Verification items for the finished model (mm, model axes). Give positions to 0.01 mm unless a question says otherwise; leave off trailing zeros. Loops run counter-clockwise (first coordinate to the right, second up) from the corner with the lowest first, then second, coordinate; pieces in that order, holes last. Notation, with made-up numbers: M 76.25,86.5 L 125.25,86.5 A10 ccw 125.25,99.5 Z; hole C -20.5,-19 d4. An arc over 180 degrees is marked long. Put each result on its own line as item: value. Start each with the question number.
from build123d import *

# Parameters (mm, degrees)
SKETCH_1_W          = 7.5
SKETCH_1_H          = 150
CUT_EXTRUDE_1_DEPTH = 1


with BuildPart() as part:
    # Sketch 1 → Revolve 1 (revolve)
    with BuildSketch(Plane.XY):
        Rectangle(SKETCH_1_W, SKETCH_1_H)
    revolve(axis=Axis((3.75, 75, 0), (0, -1, 0)))

    # Sketch 2 → Cut-Extrude 1 (cut, symmetric)
    with BuildSketch(Plane.XY):
        Polygon((1.25, -18.5), (-3.75, -24), (-27.95, -24), (-27.95, 75), (-3.75, 75), (1.25, 69.5), (-3.75, 64), (1.25, 58.5), (-3.75, 53), (1.25, 47.5), (-3.75, 42), (1.25, 36.5), (-3.75, 31), (1.25, 25.5), (-3.75, 20), (1.25, 14.5), (-3.75, 9), (1.25, 3.5), (-3.75, -2), (1.25, -7.5), (-3.75, -13), align=None)
    extrude(amount=CUT_EXTRUDE_1_DEPTH, both=True, mode=Mode.SUBTRACT)


solid = part.part
Q1. Cross-section at A-A, the plane x = -1. State how many separate pieces and enclosed holes the cut face has, then the cut area to 3 significant figures.
Q2. Cross-section at B-B, the plane y = -49.5. Record the boundary of the cut face in (x, z), then the cut area to 3 significant figures.
Q3. Go/stop test with flat-tipped pins: pin 1 (4 mm diameter, centred on x = -0.5, y = 45.5, fed in from +Z); pin 2 (2.5 mm diameter, centred on x = -0.5, y = 12, fed in from -Z); pin 3 (1.5 mm diameter, centred on y = 50.5, z = -5.5, fed in from -X). Record where each tip stops, or that it passes through.
Q4. Release check for a two-part mould opening along Z. For faces 1 (the face through (-1.215, 22.788, 0.014)), 2 (the face through (4, 75, 0)) record: pulls with the +Z half, pulls with the -Z half, needs draft (parallel to the pull), parting line crosses it, or undercut.
Q5. Cross-section at D-D, the plane z = -5.5. Record the boundary of the cut face in (x, y), then the cut area to 3 significant figures.
Q6. Cross-section at C-C, the plane x = 6.75. Record the boundary of the cut face in (y, z), then the cut area to 3 significant figures.
Q7. Scan lines: L1, parallel to X at y = -28.5, z = -2.25; L2, parallel to Z at x = 1, y = -28; L3, parallel to X at y = -28, z = -2. Record each from-to range of solid material in increasing order.
Ans:
1. separate pieces: 1
1. enclosed holes: 9
1. area: 1,650 mm^2
2. outline: C 3.75,0 d15
2. area: 177 mm^2
3. pin 1: stops at z = 7.15
3. pin 2: stops at z = -6.87
3. pin 3: stops at x = -2.05
4. face 1: undercut
4. face 2: needs draft
5. outline: M -1.35,-75 L 8.85,-75 L 8.85,75 L -1.35,75 Z
5. area: 1,530 mm^2
6. outline: M -75,-6.87 L 75,-6.87 L 75,6.87 L -75,6.87 Z
6. area: 2,060 mm^2
7. L1: x = -3.4 to 10.9
7. L2: z = -6.98 to 6.98
7. L3: x = -3.48 to 10.98
